CAD build for the part. Positions are in the model's coordinates, mm. Give positions to 0.01 mm unless a question says otherwise; leave off trailing zeros. Loops run counter-clockwise (first coordinate to the right, second up) from the corner with the lowest first, then second, coordinate; pieces in that order, holes last. Notation, with made-up numbers: M 85,-26 L 111,-26 A25 ccw 111,-5 Z; hole C 4,31.25 d7. An arc over 180 degrees is marked long. Answer as CSV lines item,"result".
```python
from build123d import *

# Parameters (mm, degrees)
SKETCH1_W                = 6.5
SKETCH1_H                = 5
BOSS_EXTRUDE1_DEPTH      = 0.75
M2_CLEARANCE_HOLE1_D     = 2.4
M2_CLEARANCE_HOLE1_DEPTH = 1.6
M2_CLEARANCE_HOLE1_TIP   = 0.721032743
FILLET1_R                = 0.1


with BuildPart() as part:
    # Sketch1 → Boss-Extrude1 (new body)
    with BuildSketch(Plane(origin=(0, 0, 0), x_dir=(1, 0, 0), z_dir=(0, 1, 0))):
        Rectangle(SKETCH1_W, SKETCH1_H)
    extrude(amount=BOSS_EXTRUDE1_DEPTH)

    # M2 Clearance Hole1
    with Locations(Plane(origin=(0, 0.75, 0), x_dir=(1, 0, 0), z_dir=(0, 1, 0))):
        with Locations((0, 0)):
            Hole(M2_CLEARANCE_HOLE1_D / 2, depth=M2_CLEARANCE_HOLE1_DEPTH)
            with Locations((0, 0, -(M2_CLEARANCE_HOLE1_DEPTH + M2_CLEARANCE_HOLE1_TIP / 2))):  # 118° drill point
                Cone(0, M2_CLEARANCE_HOLE1_D / 2, M2_CLEARANCE_HOLE1_TIP, mode=Mode.SUBTRACT)

    # Fillet1
    fillet1_edges = [part.edges().sort_by_distance(p)[0] for p in [
        (3.25, 0.75, 0),
        (0, 0.75, -2.5),
        (-3.25, 0.75, 0),
        (0, 0, -2.5),
        (3.25, 0, 0),
        (0, 0, 2.5),
        (-3.25, 0, 0),
        (-3.25, 0.375, -2.5),
        (3.25, 0.375, -2.5),
        (3.25, 0.375, 2.5),
        (-3.25, 0.375, 2.5),
        (0, 0.75, 2.5),
    ]]
    fillet(fillet1_edges, radius=FILLET1_R)


solid = part.part
```
Q1. Cut at A-A (x = 0). Write the cut outline in (y, z), and give its area (3 significant figures).
Solution:
outline,"M 0,-2.4 A0.1 ccw 0.1,-2.5 L 0.65,-2.5 A0.1 ccw 0.75,-2.4 L 0.75,-1.2 L 0,-1.2 Z; M 0,1.2 L 0.75,1.2 L 0.75,2.4 A0.1 ccw 0.65,2.5 L 0.1,2.5 A0.1 ccw 0,2.4 Z"
area,"1.94 mm²"
Q2. Cut at C-C (y = 0.2). Write the cut outline in (x, z).
Solution:
outline,"M -3.25,-2.4 A0.1 ccw -3.15,-2.5 L 3.15,-2.5 A0.1 ccw 3.25,-2.4 L 3.25,2.4 A0.1 ccw 3.15,2.5 L -3.15,2.5 A0.1 ccw -3.25,2.4 Z; hole C 0,0 d2.4"
Q3. Cut at B-B (z = 0). Write the cut outline in (x, y).
Solution:
outline,"M -3.25,0.1 A0.1 ccw -3.15,0 L -1.2,0 L -1.2,0.75 L -3.15,0.75 A0.1 ccw -3.25,0.65 Z; M 1.2,0 L 3.15,0 A0.1 ccw 3.25,0.1 L 3.25,0.65 A0.1 ccw 3.15,0.75 L 1.2,0.75 Z"
Q4. Mould opens along Z. For faces 1 (the flat face through (-1, 0, -1)), 2 (the cylindrical face through (-0.65, 0.37, -1.01)) say: released by +Z, released by -Z, zero draft, split by the parting line, or undercut.
Solution:
face 1,"zero draft"
face 2,"undercut"
Q5. Wall check: line 1 (Z direction, x = 0, y = 0.45); line 2 (Z direction, x = 1, y = 0.45); line 3 (X direction, y = 0.3, z = 0.3). Give the ranges that are in metal, low to high. Write a range as [from, to].
Solution:
line 1,"z = [-2.5, -1.2], [1.2, 2.5]"
line 2,"z = [-2.5, -0.66], [0.66, 2.5]"
line 3,"x = [-3.25, -1.16], [1.16, 3.25]"
